Design review of the part built by this model. Coordinates are the model's own, in mm. A direction names the side the tool comes from. Give positions to 0.01 mm unless a question says otherwise; leave off trailing zeros. Write each loop counter-clockwise with the first axis right and the second up, starting at its lowest first coordinate (ties: lowest second). Pieces come first, ordered by that corner, then holes. Notation, with made-up numbers: M 71,-32.75 L 113,-32.75 A34 cw 113,0.25 Z; hole C -20.75,-26 d5. An arc over 180 degrees is marked long. Use a Markdown table: item, result. Add a question column.
```python
from build123d import *

# Parameters (mm, degrees)
F0_R     = 58
F1_DEPTH = 30
F2_T     = -3
F3_R     = 2
F5_D     = 14
F7_D     = 5


with BuildPart() as f1:
    # F0 (on Front) → F1 (new body)
    with BuildSketch(Plane.XZ):
        Circle(F0_R)
    extrude(amount=F1_DEPTH)

    # F2
    f2_openings = [f1.faces().sort_by_distance(p)[0] for p in [
        (0, 0, 0),
    ]]
    offset(amount=F2_T, openings=f2_openings)

    # F3
    f3_edges = [f1.edges().sort_by_distance(p)[0] for p in [
        (-58, -30, 0),
    ]]
    fillet(f3_edges, radius=F3_R)

    # F5 (through all)
    with Locations(Plane.XZ.offset(30)):
        with Locations((0, 0)):
            Hole(F5_D / 2)

    # F7 (through all)
    with Locations(Plane.XZ.offset(30)):
        with Locations((0, 25), (0, 50), (-23.776413, 7.725425), (-47.552826, 15.45085), (-29.389263, -40.45085), (-14.694631, -20.225425), (14.694631, -20.225425), (29.389263, -40.45085), (23.776413, 7.725425), (47.552826, 15.45085)):
            Hole(F7_D / 2)


solid = f1.part
```
(1) Wall thickness on L1, parallel to Z at x = -30, y = -20.5; L2, parallel to Z at x = 25, y = -1; L3, parallel to X at y = -9.5, z = 47.5: over which ranges is each line inside the solid? List them lowest first.
(2) For pin 1 (6 mm diameter, centred on x = 29.5, y = -6, fed in from -Z); pin 2 (2 mm diameter, centred on y = -21.5, z = -10, fed in from +X); pin 3 (4.5 mm diameter, centred on x = 29.39, z = -40.45, fed in from -Y); pin 4 (4 mm diameter, centred on x = -4.5, z = 24.5, fed in from +Y), all flat-tipped, find the tip position at first contact; note any pin that passes through.
(3) Add section C-C on y = -19. Give the boundary of the cut face in (x, z).
(4) Add section B-B on x = 0. Give the boundary of the cut face in (y, z).
(5) Add section A-A on z = 0. Give the boundary of the cut face in (x, y).
(6) Machinability: for faces 4 (the flat face through (-1, -27, -11)), 5 (the cylindrical face through (22.43, -28.48, 9.83)), which of the approach directions +Z, -Z, +X, -X, +Y, -Y give a long, thin tool a straight path to every point of the face, cutting with its end or side? Answer none if there is none.
(7) The part is to be moulded in two halves that separate along Z. For faces 1 (the cylindrical face through (26.76, -13.8, -51.46)), 2 (the cylindrical face through (-11.923, -13.311, -53.692)), 3 (the flat face through (-1, -30, -12)), say which applies: released by +Z, released by -Z, zero draft, split by the parting line, or undercut.
From the geometry:
| question | item | result |
|---|---|---|
| 1 | L1 | z = -49.64 to -46.1, 46.1 to 49.64 |
| 1 | L2 | z = -52.34 to -48.99, 48.99 to 52.34 |
| 1 | L3 | x = -33.28 to -27.73, 27.73 to 33.28 |
| 2 | pin 1 | stops at z = -51.59 |
| 2 | pin 2 | stops at x = 57.3 |
| 2 | pin 3 | passes through |
| 2 | pin 4 | stops at y = -27 |
| 3 | outline | C 0,0 d116; hole C 0,0 d110 |
| 4 | outline | M -30,-56 A2 ccw -28,-58 L 0,-58 L 0,-55 L -27,-55 L -27,-7 L -30,-7 Z; M -30,7 L -27,7 L -27,22.5 L -30,22.5 Z; M -30,27.5 L -27,27.5 L -27,47.5 L -30,47.5 Z; M -30,52.5 L -27,52.5 L -27,55 L 0,55 L 0,58 L -28,58 A2 ccw -30,56 Z |
| 5 | outline | M -58,-28 A2 ccw -56,-30 L -7,-30 L -7,-27 L -55,-27 L -55,0 L -58,0 Z; M 7,-30 L 56,-30 A2 ccw 58,-28 L 58,0 L 55,0 L 55,-27 L 7,-27 Z |
| 6 | face 4 | +Y |
| 6 | face 5 | +Y, -Y |
| 7 | face 1 | split by the parting line |
| 7 | face 2 | undercut |
| 7 | face 3 | zero draft |
